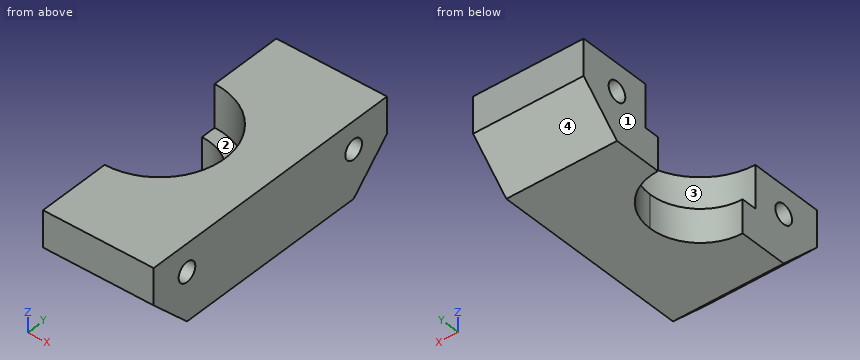
```python
from build123d import *

# Parameters (mm, degrees)
F0_W     = 35
F0_H     = 9.6
F1_DEPTH = 14
F2_R     = 8.25
F2_R_2   = 6.35
F3_DEPTH = 5.4
F4_DEPTH = 25
F5_SIZE  = 5
F7_D     = 2.5


with BuildPart() as f1:
    # F0 (on Right) → F1 (new body)
    with BuildSketch(Plane.YZ):
        Rectangle(F0_W, F0_H)
    extrude(amount=F1_DEPTH)

    # F2 (on face) → F3 (cut)
    with BuildSketch(Plane.XY.offset(4.8)):
        Circle(F2_R)
        Circle(F2_R_2, mode=Mode.SUBTRACT)
        with BuildLine():
            Line((0, -6.35), (0, 6.35))
            ThreePointArc((0, 6.35), (-6.35, 0), (0, -6.35))
        make_face()
        with BuildLine():
            ThreePointArc((0, -6.35), (4.4901280605, -4.4901280605), (6.35, 0))
            ThreePointArc((6.35, 0), (4.4901280605, 4.4901280605), (0, 6.35))
            Line((0, 6.35), (0, -6.35))
        make_face()
    extrude(amount=-F3_DEPTH, mode=Mode.SUBTRACT)

    # F2 (on face) → F4 (cut)
    with BuildSketch(Plane.XY.offset(4.8)):
        with BuildLine():
            ThreePointArc((0, -6.35), (4.4901280605, -4.4901280605), (6.35, 0))
            ThreePointArc((6.35, 0), (4.4901280605, 4.4901280605), (0, 6.35))
            Line((0, 6.35), (0, -6.35))
        make_face()
    extrude(amount=-F4_DEPTH, mode=Mode.SUBTRACT)

    # F5
    f5_edges = [f1.edges().sort_by_distance(p)[0] for p in [
        (7, 17.5, -4.8),
        (7, -17.5, -4.8),
    ]]
    chamfer(f5_edges, length=F5_SIZE)

    # F7 (through all)
    with Locations(Plane.YZ.offset(14)):
        with Locations((-12.5, 1.3), (12.5, 1.3)):
            Hole(F7_D / 2)


solid = f1.part
```
Check sheet for the modelled part. Datum: model origin and axes. Units: mm. Face numbers are marked on the shaded views. Coordinates: 2 decimals unless noted, no trailing zeros. Loops run counter-clockwise (first coordinate to the right, second up) from the corner with the lowest first, then second, coordinate; pieces in that order, holes last.
1) Release check for a two-part mould opening along Y. For the marked faces 1, 2, 3 and 4 record: released by +Y, released by -Y, zero draft, split by the parting line, or undercut.
2) Sectioned sample at A-A (z = 1.3). Record the boundary of the cut face in (x, y), and give its area (3 significant figures).
3) Sectioned sample at B-B (x = 5.75). Record the boundary of the cut face in (y, z), and give its area (3 significant figures).
4) Sectioned sample at D-D (y = 2). Record the boundary of the cut face in (x, z), and give its area (3 significant figures).
5) Sectioned sample at C-C (z = -1). Record the boundary of the cut face in (x, y).
6) Gauge pin test, flat ends, axial feed: pin 1 (5 mm diameter, centred on x = 12.5, z = -3.5, fed in from -Y); pin 2 (1.5 mm diameter, centred on y = -12.5, z = 1.3, fed in from +X). Record the tip position at first contact, or that the pin passes through.
7) Material ranges on probe 1 along Z at (x, y) = (8.5, 12.5); probe 2 along Y at (x, z) = (12, 0.25); probe 3 along Y at (x, z) = (1.25, 0.75), recorded low to high.
Check sheet entries:
1. face 1: zero draft
1. face 2: undercut
1. face 3: undercut
1. face 4: released by +Y
2. outline: (0, -17.5) - (14, -17.5) - (14, -13.75) - (0, -13.75) - close; (0, -11.25) - (14, -11.25) - (14, 11.25) - (0, 11.25) - (0, 8.25) arc R8.25 cw to (0, -8.25) - close; (0, 13.75) - (14, 13.75) - (14, 17.5) - (0, 17.5) - close
2. area: 313 mm2
3. outline: (-17.5, 0.2) - (-12.5, -4.8) - (-2.69, -4.8) - (-2.69, -0.6) - (-5.92, -0.6) - (-5.92, 4.8) - (-17.5, 4.8) - close; (2.69, -4.8) - (12.5, -4.8) - (17.5, 0.2) - (17.5, 4.8) - (5.92, 4.8) - (5.92, -0.6) - (2.69, -0.6) - close; hole circle Ø2.5 at (-12.5, 1.3); hole circle Ø2.5 at (12.5, 1.3)
3. area: 215 mm2
4. outline: (6.03, -4.8) - (14, -4.8) - (14, 4.8) - (8, 4.8) - (8, -0.6) - (6.03, -0.6) - close
4. area: 65.9 mm2
5. outline: (0, -16.3) - (14, -16.3) - (14, 16.3) - (0, 16.3) - (0, 6.35) arc R6.35 cw to (0, -6.35) - close
6. pin 1: stops at y = -16.3
6. pin 2: passes through
7. probe 1: z = -4.8 to 0.05, 2.55 to 4.8
7. probe 2: y = -17.5 to -13.18, -11.82 to 11.82, 13.18 to 17.5
7. probe 3: y = -17.5 to -13.62, -11.38 to -8.15, 8.15 to 11.38, 13.62 to 17.5
